```python
from build123d import *

# Parameters (mm, degrees)
F1_DEPTH      = 22
F1_DEPTH_BACK = 22
F2_SIZE       = 2
F3_R          = 2.25
F4_DEPTH      = 10


with BuildPart() as f1:
    # F0 (on Front) → F1 (new body, two sides)
    with BuildSketch(Plane.XZ) as f1_sk:
        Polygon((22, -22), (22, 22), (-4, 22), (-4, 0), (-22, 0), (-22, -22), align=None)
    extrude(amount=F1_DEPTH)
    extrude(f1_sk.sketch, amount=-F1_DEPTH_BACK)

    # F2
    f2_edges = [f1.edges().sort_by_distance(p)[0] for p in [
        (22, 0, 22),
        (9, -22, 22),
        (9, 22, 22),
        (22, 22, 0),
        (22, -22, 0),
        (-22, -22, -11),
        (-22, 22, -11),
        (22, 0, -22),
        (0, 22, -22),
        (0, -22, -22),
        (-22, 0, -22),
    ]]
    chamfer(f2_edges, length=F2_SIZE)

    # F3 (on face) → F4 (cut)
    with BuildSketch(Plane(origin=(0, 0, -22), x_dir=(1, 0, 0), z_dir=(0, 0, -1))):
        with Locations((-16, 16)):
            Circle(F3_R)
        with Locations((16, 16)):
            Circle(F3_R)
        with Locations((16, -16)):
            Circle(F3_R)
        with Locations((-16, -16)):
            Circle(F3_R)
    extrude(amount=-F4_DEPTH, mode=Mode.SUBTRACT)


solid = f1.part
```
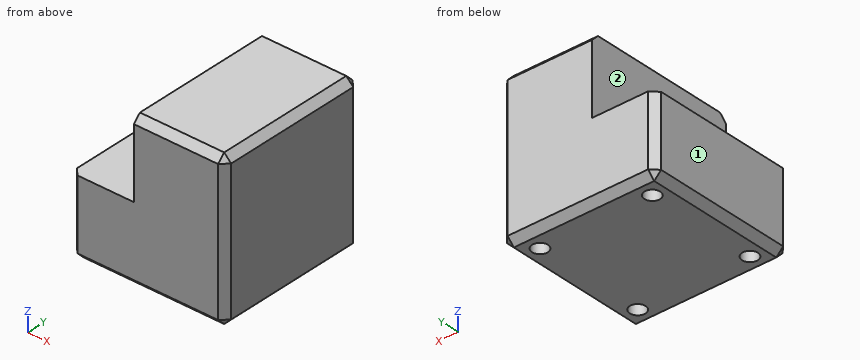
Build history of the part. All positions in model axes, mm. Face numbers are marked on the shaded views. A direction names the side the tool comes from. Round coordinates to 2 decimals unless told otherwise and drop trailing zeros. Write each loop counter-clockwise with the first axis right and the second up, starting at its lowest first coordinate (ties: lowest second). Pieces come first, ordered by that corner, then holes. Notation, with made-up numbers: (9, 31.25) - (19, 31.25) arc R20 cw to (19, 40.25) - close; hole circle Ø3 at (-23.75, 17). An arc over 180 degrees is marked (long way). Write each question's results on one line, items separated by ' | '. Start each with the question number.
Item 1: Saw through at C-C (x = -10). Write the cut outline in (y, z).
Item 2: Wall check: L1, parallel to X at y = -16, z = -17; L2, parallel to Z at x = -13.5, y = 12. Give the ranges that are in metal, low to high. Write a range as [from, to].
Item 3: Which spindle directions (+Z, -Z, +X, -X, +Y, -Y) get a long thin tool onto all of the face, cutting with end or side? Do the marked faces 1 and 2. Say none if no direction does.
Item 4: Saw through at D-D (z = 16.5). Write the cut outline in (x, y), and give its area (3 significant figures).
Item 5: Saw through at A-A (z = -16). Write the cut outline in (x, y).
Item 6: Saw through at B-B (y = -16). Write the cut outline in (x, z).
Item 7: Drop flat-ended pins along their axis: P1, Ø7, axis at x = -16, y = 16, coming from the +Z side; P2, Ø8, axis at x = -7.5, z = 2, coming from the -Y side; P3, Ø3.5, axis at x = -16, y = -16, coming from the -Z side; P4, Ø6, axis at y = 15, z = 9.5, coming from the -X side. Give the stop position or say it passes through.
Results are:
1) outline: (-22, -20) - (-20, -22) - (20, -22) - (22, -20) - (22, 0) - (-22, 0) - close
2) L1: x = [-22, -18.25], [-13.75, 13.75], [18.25, 22] | L2: z = [-22, 0]
3) face 1: +Z, -Z, -X, +Y, -Y | face 2: +Z, -X, +Y, -Y
4) outline: (-4, -22) - (20, -22) - (22, -20) - (22, 20) - (20, 22) - (-4, 22) - close | area: 1,140 mm²
5) outline: (-22, -20) - (-20, -22) - (20, -22) - (22, -20) - (22, 20) - (20, 22) - (-20, 22) - (-22, 20) - close; hole circle Ø4.5 at (-16, -16); hole circle Ø4.5 at (-16, 16); hole circle Ø4.5 at (16, -16); hole circle Ø4.5 at (16, 16)
6) outline: (-22, -20) - (-20, -22) - (-18.25, -22) - (-18.25, -12) - (-13.75, -12) - (-13.75, -22) - (13.75, -22) - (13.75, -12) - (18.25, -12) - (18.25, -22) - (20, -22) - (22, -20) - (22, 20) - (20, 22) - (-4, 22) - (-4, 0) - (-22, 0) - close
7) P1: stops at z = 0 | P2: stops at y = -22 | P3: stops at z = -12 | P4: stops at x = -4
